The listing builds one solid part. Answer for the finished solid, in the listing's coordinates (mm). Give positions to 0.01 mm unless a question says otherwise; leave off trailing zeros. Loops run counter-clockwise (first coordinate to the right, second up) from the corner with the lowest first, then second, coordinate; pieces in that order, holes last. Notation, with made-up numbers: (-16, 30.5) -> (0, 30.5) arc R14 cw to (0, 55.5) -> close; hole circle Ø6 at (7.5, -2). An arc over 180 degrees is marked (long way). One line per question, with ' | ' between items. Start each with the question number.
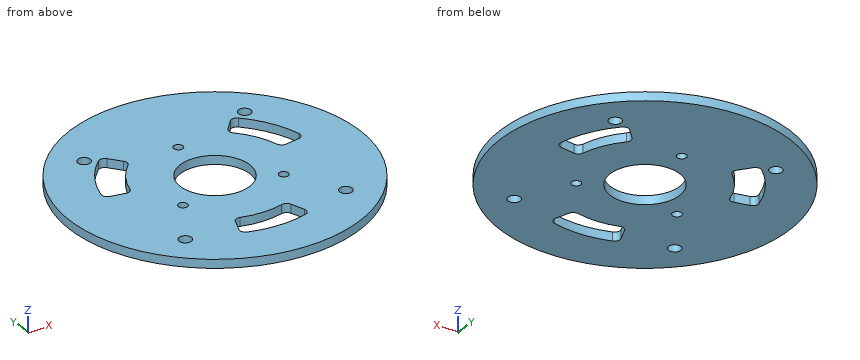
from build123d import *

# Parameters (mm, degrees)
SKETCH_1_R                       = 50
SKETCH_1_R_2                     = 12
EXTRUDE_1_DEPTH                  = 3
SKETCH_2_R                       = 1.6
CUT_EXTRUDE_1_DEPTH              = 71.774289117
CUT_EXTRUDE_3_DEPTH              = 71.774289117
FILLET_1_R                       = 2
PATTERN_CIRCULAR_2_COUNT         = 3
FILLET_1_OF_PATTERN_CIRCULAR_2_R = 2
SKETCH_5_R                       = 2.15
CUT_EXTRUDE_4_DEPTH              = 10


with BuildPart() as part:
    # 草图1 → 凸台-拉伸1 (new body)
    with BuildSketch(Plane.XY):
        Circle(SKETCH_1_R)
        Circle(SKETCH_1_R_2, mode=Mode.SUBTRACT)
    extrude(amount=EXTRUDE_1_DEPTH)

    # 草图2 → 切除-拉伸1 (cut, through all)
    with BuildSketch(Plane.XY.offset(3)):
        with Locations((0.263678953, 19.99826176)):
            Circle(SKETCH_2_R)
        with Locations((17.187163239, -10.227483551)):
            Circle(SKETCH_2_R)
        with Locations((-17.450842192, -9.770778208)):
            Circle(SKETCH_2_R)
    extrude(amount=-CUT_EXTRUDE_1_DEPTH, mode=Mode.SUBTRACT)

    # 草图4 → 切除-拉伸3 (cut, through all)
    with BuildSketch(Plane(origin=(0, 0, 0), x_dir=(-1, 0, 0), z_dir=(0, 0, -1))):
        with BuildLine():
            Line((16.448438601, 20.135760914), (22.142128886, 27.105831999))
            ThreePointArc((22.142128886, 27.105831999), (30.077535668, 17.898096215), (34.385147752, 6.531585879))
            Line((34.385147752, 6.531585879), (25.543252616, 4.852035224))
            ThreePointArc((25.543252616, 4.852035224), (22.343312211, 13.295728617), (16.448438601, 20.135760914))
        make_face()
    cut_extrude_3 = extrude(amount=-CUT_EXTRUDE_3_DEPTH, mode=Mode.SUBTRACT)

    # 圆角1
    fillet_1_edges = [part.edges().sort_by_distance(p)[0] for p in [
        (-25.543252616, 4.852035224, 1.5),
        (-16.448438601, 20.135760914, 1.5),
        (-22.142128886, 27.105831999, 1.5),
        (-34.385147752, 6.531585879, 1.5),
    ]]
    fillet(fillet_1_edges, radius=FILLET_1_R)

    # 阵列(圆周)2: 切除-拉伸3 ×3 about axis
    pattern_circular_2_axis = Axis((0, 0, 0), (0, 0, 1))
    for i in range(1, PATTERN_CIRCULAR_2_COUNT):
        add(cut_extrude_3.rotate(pattern_circular_2_axis, i * 360 / PATTERN_CIRCULAR_2_COUNT), mode=Mode.SUBTRACT)

    # 圆角1 of 阵列(圆周)2
    fillet_1_of_pattern_circular_2_edges = [part.edges().sort_by_distance(p)[0] for p in [
        (8.569640543, -24.547123273, 1.5),
        (-9.213861175, -24.312646138, 1.5),
        (-12.403274659, -32.728562109, 1.5),
        (11.536054578, -33.044204405, 1.5),
        (16.973612072, 19.695088048, 1.5),
        (25.662299777, 4.176885224, 1.5),
        (34.545403545, 5.62273011, 1.5),
        (22.849093174, 26.512618526, 1.5),
    ]]
    fillet(fillet_1_of_pattern_circular_2_edges, radius=FILLET_1_OF_PATTERN_CIRCULAR_2_R)

    # 草图5 → 切除-拉伸4 (cut)
    with BuildSketch(Plane.XY):
        with Locations((27.938343572, 27.211191787)):
            Circle(SKETCH_5_R)
        with Locations((27.211191787, -27.938343572)):
            Circle(SKETCH_5_R)
        with Locations((-27.938343572, -27.211191787)):
            Circle(SKETCH_5_R)
        with Locations((-27.211191787, 27.938343572)):
            Circle(SKETCH_5_R)
    extrude(amount=CUT_EXTRUDE_4_DEPTH, mode=Mode.SUBTRACT)


solid = part.part
1. Straight lines are drawn through the part: L1, parallel to X at y = 19, z = 2.1; L2, parallel to Y at x = -28, z = 1.35; L3, parallel to X at y = 27, z = 0.8. For each, find the intervals that lie inside material, in ascending order.
2. The part is cut by section B-B (x = 20). Write down the section's boundary in (y, z), plus the area to 3 significant figures.
3. The part is cut by section D-D (x = 0). Write down the section's boundary in (y, z), plus the area to 3 significant figures.
4. The part is cut by section C-C (y = 23). Write down the section's boundary in (x, z), plus the area to 3 significant figures.
5. Each of these flat-tipped pins is pushed along its axis until it touches: pin 1 Ø21.5 at (x, y) = (0, 0) entering from -Z; pin 2 Ø1 at (y, z) = (6, 1) entering from +X; pin 3 Ø1 at (x, z) = (33, 2.5) entering from -Y. Where does it stop, or does it pass through?
6. The part is cut by section A-A (y = 0). Write down the section's boundary in (x, z), plus the area to 3 significant figures.
Check sheet entries:
1) L1: x = -46.25 to -29.39, -17.75 to -0.99, 1.51 to 17.94, 29.39 to 46.25 | L2: y = -41.42 to -29.36, -25.06 to 5.32, 21 to 25.94, 29.94 to 41.42 | L3: x = -42.08 to -29.15, -25.28 to 25.8, 30.08 to 42.08
2) outline: (-45.83, 0) -> (16.61, 0) -> (16.61, 3) -> (-45.83, 3) -> close; (23.21, 0) -> (45.83, 0) -> (45.83, 3) -> (23.21, 3) -> close | area: 255 mm^2
3) outline: (-50, 0) -> (-35, 0) -> (-35, 3) -> (-50, 3) -> close; (-26, 0) -> (-12, 0) -> (-12, 3) -> (-26, 3) -> close; (12, 0) -> (18.42, 0) -> (18.42, 3) -> (12, 3) -> close; (21.58, 0) -> (50, 0) -> (50, 3) -> (21.58, 3) -> close | area: 192 mm^2
4) outline: (-44.4, 0) -> (-26.38, 0) -> (-26.38, 3) -> (-44.4, 3) -> close; (-18.79, 0) -> (19.82, 0) -> (19.82, 3) -> (-18.79, 3) -> close; (26.38, 0) -> (44.4, 0) -> (44.4, 3) -> (26.38, 3) -> close | area: 224 mm^2
5) pin 1: passes through | pin 2: stops at x = 49.7 | pin 3: stops at y = -38
6) outline: (-50, 0) -> (-12, 0) -> (-12, 3) -> (-50, 3) -> close; (12, 0) -> (50, 0) -> (50, 3) -> (12, 3) -> close | area: 228 mm^2
